Solid Edge part; units mm, degrees
sketch "Sketch1" plane through (0, 0, 0) normal (0, 0, 1) x (1, 0, 0)
  line L0 (-15, 5.75) -> (15, 5.75)
  line L1 (15, 5.75) -> (15, -5.75)
  line L2 (15, -5.75) -> (-15, -5.75)
  line L3 (-15, -5.75) -> (-15, 5.75)
  dimension "D1" = 15
  dimension "D2" = 15
extrude "Protrusion1" add sketch "Sketch1" along normal blind 2
fillet "Avrundningar_1" radius 1 4 edges at (-15, -5.75, 1) (15, -5.75, 1) (15, 5.75, 1) (-15, 5.75, 1)
sketch "Sketch2" plane through (0, 0, 2) normal (0, 0, 1) x (0, 1, 0)
  circle A0 centre (-2.75, 12) radius 1.5598
  circle A1 centre (2.75, 12) radius 1.5598
  circle A2 centre (-2.75, -12) radius 1.5598
  circle A3 centre (2.75, -12) radius 1.5598
  dimension "D1" = 2.75
  dimension "D2" = 2.75
extrude "Försänkningar_för_fjäder" cut sketch "Sketch2" against normal blind 1
The model under review builds one solid part; all positions refer to its coordinate system, in mm. A direction names the side the tool comes from. Round coordinates to 2 decimals unless told otherwise and drop trailing zeros. Loops run counter-clockwise (first coordinate to the right, second up) from the corner with the lowest first, then second, coordinate; pieces in that order, holes last. Notation, with made-up numbers: M -15.75,51 L 28.25,51 A19 cw 28.25,79 Z; hole C 1,25 d6. An arc over 180 degrees is marked long. Answer as a JSON object with one key per item and string values.
Item 1: The part is to be moulded in two halves that separate along X. For faces 1 (the face through (-15, 0, 1)), 2 (the face through (14.699, -5.465, 1.014)), 3 (the face through (10.685, -1.911, 1.507)), say which applies: +X half, -X half, draft (parallel to the pull), parting line (faces both ways), or undercut.
Check sheet entries:
{"face 1": "-X half", "face 2": "+X half", "face 3": "undercut"}
Item 2: We need section A-A, the plane z = 1.6. State the section outline as (x, y) points.
Check sheet entries:
{"outline": "M -15,-4.75 A1 ccw -14,-5.75 L 14,-5.75 A1 ccw 15,-4.75 L 15,4.75 A1 ccw 14,5.75 L -14,5.75 A1 ccw -15,4.75 Z; hole C -12,-2.75 d3.12; hole C -12,2.75 d3.12; hole C 12,-2.75 d3.12; hole C 12,2.75 d3.12"}
Item 3: Tool access review of faces 4 (the face through (0, -5.75, 1)), 5 (the face through (-12, 3, 1)): name each direction out of +Z, -Z, +X, -X, +Y, -Y from which nothing blocks a thin tool from reaching the whole face with its end or side.
Check sheet entries:
{"face 4": "+Z, -Z, +X, -X, -Y", "face 5": "+Z"}
Item 4: We need section C-C, the plane x = 12. State the section outline as (y, z) points.
Check sheet entries:
{"outline": "M -5.75,0 L 5.75,0 L 5.75,2 L 4.31,2 L 4.31,1 L 1.19,1 L 1.19,2 L -1.19,2 L -1.19,1 L -4.31,1 L -4.31,2 L -5.75,2 Z"}
Item 5: Clearance check with a flat-ended pin moving along its axis: P1, Ø0.9, axis at x = 12.5, y = -3.5, coming from the +Z side. State where the tip first meets the part, or that it passes through.
Check sheet entries:
{"P1": "z = 1"}
Item 6: For line 1 along Y through (x, z) = (12, 1.75); line 2 along X through (y, z) = (2.75, 1.75); line 3 along Y through (x, z) = (11.5, 1.85), list the stretches that pass through material, from the lowest coordinate up.
Check sheet entries:
{"line 1": "-5.75 to -4.31, -1.19 to 1.19, 4.31 to 5.75", "line 2": "-15 to -13.56, -10.44 to 10.44, 13.56 to 15", "line 3": "-5.75 to -4.23, -1.27 to 1.27, 4.23 to 5.75"}
Item 7: We need section B-B, the plane y = -2.75. State the section outline as (x, z) points.
Check sheet entries:
{"outline": "M -15,0 L 15,0 L 15,2 L 13.56,2 L 13.56,1 L 10.44,1 L 10.44,2 L -10.44,2 L -10.44,1 L -13.56,1 L -13.56,2 L -15,2 Z"}
